For this review, take the finished solid that the model builds, in its own axes (mm). A direction names the side the tool comes from. Give positions to 0.01 mm unless a question says otherwise; leave off trailing zeros. Write each loop counter-clockwise with the first axis right and the second up, starting at its lowest first coordinate (ties: lowest second). Pieces come first, ordered by that corner, then holes.
Q1. Insertion check: P1, Ø7.5, axis at x = -19.05, y = 9.525, coming from the -Z side; P2, Ø3, axis at y = -20.5, z = -1.5, coming from the +X side; P3, Ø5, axis at x = 22, z = -8, coming from the -Y side; P4, Ø1, axis at y = -22.5, z = -3, coming from the -X side. Each pin has a flat end and moves straight along its axis. Give the tip position at first contact, or say it passes through.
Q2. For line 1 (X direction, y = 9.5, z = 5); line 2 (X direction, y = 11, z = 10); line 3 (Z direction, x = 4, y = 6), list the stretches that pass through material, from the lowest coordinate up.
Q3. Machinability: for faces 4 (the flat face through (-0.356, 22.269, 13.545)), 5 (the flat face through (-22, 0, 10)), 6 (the flat face through (0, -39.959, 12)), which of the approach directions +Z, -Z, +X, -X, +Y, -Y give a long, thin tool a straight path to every point of the face, cutting with its end or side? Answer none if there is none.
Q4. We need section B-B (z = 14.5). Write out the cut boundary in (x, y) (3 decimals).
Q5. Mouldability with a two-part tool opening along X and no side actions: class faces 1 (the flat face through (22, 0, -11)), 2 (the flat face through (15.83, -3.22, -10.5)), 3 (the cylindrical face through (16.8, 10.4, 10.5)) as released by +X, released by -X, zero draft, split by the parting line, or undercut.
Q6. We need section C-C (y = 21). Write out the cut boundary in (x, z).
Q7. We need section D-D (x = 10.5). Write out the cut boundary in (y, z).
Q8. We need section A-A (x = -14). Write out the cut boundary in (y, z).
```python
from build123d import *

# Parameters (mm, degrees)
SKETCH1_W             = 25.4
SKETCH1_H             = 12.7
BOSS_EXTRUDE1_DEPTH   = 25.4
BOSS_EXTRUDE1_2_DEPTH = 25.4
SKETCH1_3_W           = 25.4
SKETCH1_3_H           = 8.128
SKETCH1_3_H_2         = 12.7
BOSS_EXTRUDE2_DEPTH   = 43.184694682
SKETCH2_W             = 25.4
SKETCH2_H             = 3.2258
CUT_EXTRUDE1_DEPTH    = 10.16
CHAMFER1_SIZE         = 6.35
BOSS_EXTRUDE3_DEPTH   = 12.7
CUT_EXTRUDE3_DEPTH    = 34.528
CHAMFER2_SIZE         = 6.35


with BuildPart() as part:
    # Sketch1 → Boss-Extrude1 (new body)
    with BuildSketch(Plane(origin=(0, 0, 0), x_dir=(1, 0, 0), z_dir=(0, 1, 0))):
        with Locations((0, 10.414)):
            Rectangle(SKETCH1_W, SKETCH1_H)
    extrude(amount=BOSS_EXTRUDE1_DEPTH)



with BuildPart() as body_2:
    # Sketch1 → Boss-Extrude1 2 (new body)
    with BuildSketch(Plane(origin=(0, 0, 0), x_dir=(1, 0, 0), z_dir=(0, 1, 0))):
        with Locations((0, -10.414)):
            Rectangle(SKETCH1_W, SKETCH1_H)
    extrude(amount=BOSS_EXTRUDE1_2_DEPTH)


with BuildPart() as part_1:
    add(part.part)

    add(body_2.part)  # Boss-Extrude2 merges body 2
    # Sketch1_3 → Boss-Extrude2 (add)
    with BuildSketch(Plane(origin=(0, 0, 0), x_dir=(1, 0, 0), z_dir=(0, 1, 0))):
        Rectangle(SKETCH1_3_W, SKETCH1_3_H)
        with Locations((0, -10.414)):
            Rectangle(SKETCH1_3_W, SKETCH1_3_H_2)
        with Locations((0, 10.414)):
            Rectangle(SKETCH1_3_W, SKETCH1_3_H_2)
    extrude(amount=-BOSS_EXTRUDE2_DEPTH)

    # Sketch2 → Cut-Extrude1 (cut)
    with BuildSketch(Plane.XY.offset(16.764)):
        with Locations((0, -41.571794682)):
            Rectangle(SKETCH2_W, SKETCH2_H)
    extrude(amount=-CUT_EXTRUDE1_DEPTH, mode=Mode.SUBTRACT)

    # Chamfer1
    chamfer1_edges = [part_1.edges().sort_by_distance(p)[0] for p in [
        (0, 25.4, -16.764),
        (0, 25.4, 16.764),
    ]]
    chamfer(chamfer1_edges, length=CHAMFER1_SIZE)

    # Sketch5 → Boss-Extrude3 (add)
    with BuildSketch(Plane.ZY.offset(12.7)):
        Polygon((-10.414, 25.4), (-16.764, 19.05), (-16.764, 0), (-4.064, 0), (-4.064, 25.4), align=None)
        Polygon((4.064, 25.4), (4.064, 0), (16.764, 0), (16.764, 19.05), (10.414, 25.4), align=None)
    boss_extrude3 = extrude(amount=BOSS_EXTRUDE3_DEPTH)

    # Mirror1: Boss-Extrude3 across plane
    add(boss_extrude3.mirror(Plane(origin=(0, 0, 0), x_dir=(0, 0, 1), z_dir=(1, 0, 0))))

    # Sketch6 → Cut-Extrude3 (cut, through all)
    with BuildSketch(Plane.XY.offset(16.764)):
        with BuildLine():
            ThreePointArc((-16.637, 9.525), (-19.05, 11.938), (-21.463, 9.525))
            Line((-21.463, 9.525), (-16.637, 9.525))
        make_face()
        with BuildLine():
            Line((-16.637, 9.525), (-21.463, 9.525))
            ThreePointArc((-21.463, 9.525), (-19.05, 7.112), (-16.637, 9.525))
        make_face()
        with BuildLine():
            ThreePointArc((21.463, 9.525), (19.05, 11.938), (16.637, 9.525))
            Line((16.637, 9.525), (21.463, 9.525))
        make_face()
        with BuildLine():
            Line((21.463, 9.525), (16.637, 9.525))
            ThreePointArc((16.637, 9.525), (19.05, 7.112), (21.463, 9.525))
        make_face()
    extrude(amount=-CUT_EXTRUDE3_DEPTH, mode=Mode.SUBTRACT)

    # Chamfer2
    chamfer2_edges = [part_1.edges().sort_by_distance(p)[0] for p in [
        (-12.7, 0, 10.414),
        (12.7, 0, -10.414),
        (12.7, 0, 10.414),
        (-12.7, 0, -10.414),
    ]]
    chamfer(chamfer2_edges, length=CHAMFER2_SIZE)


solid = part_1.part
```
Computed:
1. P1: stops at z = -16.76
1. P2: stops at x = 12.7
1. P3: stops at y = 0
1. P4: stops at x = -12.7
2. line 1: x = -25.4 to -21.46, -16.64 to 16.64, 21.46 to 25.4
2. line 2: x = -25.4 to -20.96, -17.14 to 17.14, 20.96 to 25.4
2. line 3: z = -16.76 to -4.06, 4.06 to 16.76
3. face 4: +Z, +X, -X, +Y
3. face 5: +Z, -Z, -X, -Y
3. face 6: +Z, +X, -X, -Y
4. outline: (-25.4, 0) - (-19.05, 0) - (-12.7, -6.35) - (-12.7, -39.959) - (12.7, -39.959) - (12.7, -6.35) - (19.05, 0) - (25.4, 0) - (25.4, 21.314) - (-25.4, 21.314) - close; hole circle Ø4.826 at (-19.05, 9.525); hole circle Ø4.826 at (19.05, 9.525)
5. face 1: zero draft
5. face 2: released by +X
5. face 3: undercut
6. outline: (-25.4, -14.81) - (25.4, -14.81) - (25.4, -4.06) - (-25.4, -4.06) - close; (-25.4, 4.06) - (25.4, 4.06) - (25.4, 14.81) - (-25.4, 14.81) - close
7. outline: (-43.18, -16.76) - (19.05, -16.76) - (25.4, -10.41) - (25.4, -4.06) - (0, -4.06) - (0, 4.06) - (25.4, 4.06) - (25.4, 10.41) - (19.05, 16.76) - (-39.96, 16.76) - (-39.96, 6.6) - (-43.18, 6.6) - close
8. outline: (-5.05, -16.76) - (19.05, -16.76) - (25.4, -10.41) - (25.4, -4.06) - (-5.05, -4.06) - close; (-5.05, 4.06) - (25.4, 4.06) - (25.4, 10.41) - (19.05, 16.76) - (-5.05, 16.76) - close
